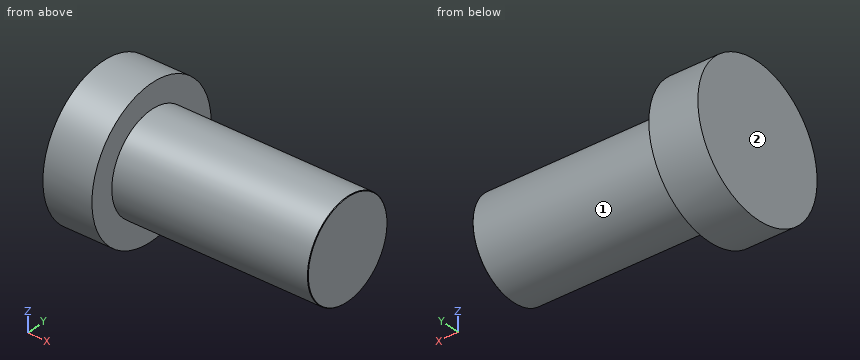
from build123d import *

# Parameters (mm, degrees)
F0_R     = 19.05
F1_DEPTH = 12.7
F2_R     = 12.7
F3_DEPTH = 50.8
F4_SIZE  = 0.127


with BuildPart() as f1:
    # F0 (on Right) → F1 (new body)
    with BuildSketch(Plane.YZ):
        Circle(F0_R)
    extrude(amount=-F1_DEPTH)

    # F2 (on face) → F3 (join)
    with BuildSketch(Plane.YZ):
        Circle(F2_R)
    extrude(amount=F3_DEPTH)

    # F4
    f4_edges = [f1.edges().sort_by_distance(p)[0] for p in [
        (50.8, -12.7, 0),
    ]]
    chamfer(f4_edges, length=F4_SIZE)


solid = f1.part
Could you check a few things on this model? Use its own coordinates, in mm. Face numbers are marked on the shaded views. A direction names the side the tool comes from. Coordinates: 2 decimals unless noted, no trailing zeros. Write each loop counter-clockwise with the first axis right and the second up, starting at its lowest first coordinate (ties: lowest second). Pieces come first, ordered by that corner, then holes. Notation, with made-up numbers: (-12.5, 24.25) - (33.5, 24.25) arc R22 cw to (33.5, 51.25) - close; hole circle Ø5 at (-29.75, 42). An arc over 180 degrees is marked (long way). Put each result on its own line as item: value. Start each with the question number.
Q1. I'm going to push flat-ended pins straight in: P1, Ø12, axis at x = 14.5, z = 0, coming from the +Y side; P2, Ø12, axis at x = -0.5, y = 8.5, coming from the +Z side; P3, Ø3, axis at x = 0.5, y = -4.5, coming from the -Z side. Where does each tip first touch, or does it pass through?
Q2. I want a section at D-D on y = -14. Write out the boundary of the cut face in (x, z).
Q3. I want a section at C-C on x = 27.5. Write out the boundary of the cut face in (y, z).
Q4. I want a section at A-A on z = 0. Write out the boundary of the cut face in (x, y), plus the area to 3 significant figures.
Q5. Which directions (+Z, -Z, +X, -X, +Y, -Y) give clear straight access to the entire face, cutting with the end or side of a thin tool? Please do the marked faces 1 and 2.
Q6. Please list where these lines run through material, in increasing order: L1, parallel to X at y = -0.5, z = -13.5; L2, parallel to Y at x = -4, z = -0.5; L3, parallel to Z at x = -1.5, y = 7.5.
Checks:
1. P1: y = 12.7
1. P2: z = 18.89
1. P3: z = -18.8
2. outline: (-12.7, -12.92) - (0, -12.92) - (0, 12.92) - (-12.7, 12.92) - close
3. outline: circle Ø25.4 at (0, 0)
4. outline: (-12.7, -19.05) - (0, -19.05) - (0, -12.7) - (50.67, -12.7) - (50.8, -12.57) - (50.8, 12.57) - (50.67, 12.7) - (0, 12.7) - (0, 19.05) - (-12.7, 19.05) - close
4. area: 1,770 mm²
5. face 1: +X
5. face 2: +Z, -Z, -X, +Y, -Y
6. L1: -12.7 to 0
6. L2: -19.04 to 19.04
6. L3: -17.51 to 17.51
